For this review, take the finished solid that the model builds, in its own axes (mm). A direction names the side the tool comes from. Round coordinates to 2 decimals unless told otherwise and drop trailing zeros. Order: outer loops, then holes, each group sorted by start corner. A loop starts at its lowest first (then second) coordinate and runs counter-clockwise, first axis right, second up. Notation, with made-up numbers: (73.5, -4.75) -> (86.5, -4.75) arc R31 cw to (86.5, 25.25) -> close; hole circle Ø3 at (-23.75, 2.5). An arc over 180 degrees is marked (long way). Answer in a Markdown table with one row per item.
```python
from build123d import *

# Parameters (mm, degrees)
CROQUIS1_W               = 16.7
CROQUIS1_H               = 20.1
SALIENTE_EXTRUIR1_DEPTH  = 3.2
CROQUIS2_W               = 20
CROQUIS2_H               = 3.2
SALIENTE_EXTRUIR2_DEPTH  = 16.7
SALIENTE_EXTRUIR3_DEPTH  = 2.2
SALIENTE_EXTRUIR4_DEPTH  = 2.2
CROQUIS5_W               = 6.7
CROQUIS5_H               = 2.4
CORTAR_EXTRUIR1_DEPTH    = 3.2
CROQUIS6_W               = 6.7
CROQUIS6_H               = 2.3
CORTAR_EXTRUIR2_DEPTH    = 3.2
CROQUIS7_W               = 4.1
CROQUIS7_H               = 1.18
SALIENTE_EXTRUIR9_DEPTH  = 1.45
SALIENTE_EXTRUIR10_DEPTH = 4.1
CROQUIS10_W              = 4.098890586
CROQUIS10_H              = 1.18
SALIENTE_EXTRUIR13_DEPTH = 1.45
SALIENTE_EXTRUIR14_DEPTH = 4.1
SALIENTE_EXTRUIR16_DEPTH = 4.1


with BuildPart() as part:
    # Croquis1 → Saliente-Extruir1 (new body)
    with BuildSketch(Plane.XY):
        Rectangle(CROQUIS1_W, CROQUIS1_H)
    extrude(amount=SALIENTE_EXTRUIR1_DEPTH)

    # Croquis2 → Saliente-Extruir2 (add)
    with BuildSketch(Plane.ZY.offset(8.35)):
        with Locations((10, 8.45)):
            Rectangle(CROQUIS2_W, CROQUIS2_H)
    extrude(amount=-SALIENTE_EXTRUIR2_DEPTH)

    # Croquis3 → Saliente-Extruir3 (add)
    with BuildSketch(Plane.ZY.offset(8.35)):
        Polygon((20, 6.85), (3.2, -10.05), (3.2, 6.85), align=None)
    extrude(amount=-SALIENTE_EXTRUIR3_DEPTH)

    # Croquis4 → Saliente-Extruir4 (add)
    with BuildSketch(Plane(origin=(8.35, 0, 0), x_dir=(0, 0, -1), z_dir=(1, 0, 0))):
        Polygon((-20, 6.85), (-3.2, -10.05), (-3.2, 6.85), align=None)
    extrude(amount=-SALIENTE_EXTRUIR4_DEPTH)

    # Croquis5 → Cortar-Extruir1 (cut)
    with BuildSketch(Plane(origin=(0, 0, 0), x_dir=(-1, 0, 0), z_dir=(0, 0, -1))):
        with BuildLine():
            ThreePointArc((-3.35, 1.5), (0, 4.85), (3.35, 1.5))
            Line((3.35, 1.5), (-3.35, 1.5))
        make_face()
        with Locations((0, 0.3)):
            Rectangle(CROQUIS5_W, CROQUIS5_H)
        with BuildLine():
            Line((3.35, -0.9), (-3.35, -0.9))
            ThreePointArc((-3.35, -0.9), (0, -4.25), (3.35, -0.9))
        make_face()
    extrude(amount=-CORTAR_EXTRUIR1_DEPTH, mode=Mode.SUBTRACT)

    # Croquis6 → Cortar-Extruir2 (cut)
    with BuildSketch(Plane(origin=(0, 10.05, 0), x_dir=(1, 0, 0), z_dir=(0, 1, 0))):
        with BuildLine():
            ThreePointArc((-3.35, -9.15), (0, -5.8), (3.35, -9.15))
            Line((3.35, -9.15), (-3.35, -9.15))
        make_face()
        with Locations((0, -10.3)):
            Rectangle(CROQUIS6_W, CROQUIS6_H)
        with BuildLine():
            Line((3.35, -11.45), (-3.35, -11.45))
            ThreePointArc((-3.35, -11.45), (0, -14.8), (3.35, -11.45))
        make_face()
    extrude(amount=-CORTAR_EXTRUIR2_DEPTH, mode=Mode.SUBTRACT)

    # Croquis7 → Saliente-Extruir9 (add)
    with BuildSketch(Plane(origin=(0, 0, 0), x_dir=(-1, 0, 0), z_dir=(0, 0, -1))):
        with Locations((0, 7.46)):
            Rectangle(CROQUIS7_W, CROQUIS7_H)
        with Locations((0, -7.34)):
            Rectangle(CROQUIS7_W, CROQUIS7_H)
    extrude(amount=SALIENTE_EXTRUIR9_DEPTH)

    # Croquis9 → Saliente-Extruir10 (add)
    with BuildSketch(Plane.ZY.offset(2.05)):
        Polygon((-1.45, 6.87), (0, 5.75), (0, 6.87), align=None)
        Polygon((-1.45, -7.93), (0, -9.05), (0, -7.93), align=None)
    extrude(amount=-SALIENTE_EXTRUIR10_DEPTH)

    # Croquis10 → Saliente-Extruir13 (add)
    with BuildSketch(Plane(origin=(0, 10.05, 0), x_dir=(1, 0, 0), z_dir=(0, 1, 0))):
        with Locations((-0.000554707, -2.59)):
            Rectangle(CROQUIS10_W, CROQUIS10_H)
        with Locations((-0.000554707, -17.29)):
            Rectangle(CROQUIS10_W, CROQUIS10_H)
    extrude(amount=SALIENTE_EXTRUIR13_DEPTH)

    # Croquis12 → Saliente-Extruir14 (add)
    with BuildSketch(Plane(origin=(2.048890586, 0, 0), x_dir=(0, 0, -1), z_dir=(1, 0, 0))):
        Polygon((-17.88, 11.5), (-19, 10.05), (-17.88, 10.05), align=None)
        Polygon((-3.18, 11.5), (-4.3, 10.05), (-3.18, 10.05), align=None)
    extrude(amount=-SALIENTE_EXTRUIR14_DEPTH)

    # Croquis13 → Saliente-Extruir16 (add)
    with BuildSketch(Plane.ZY.offset(2.05)):
        Polygon((2, 11.5), (2, 10.05), (4.3, 10.05), (3.18, 11.5), align=None)
        Polygon((16.7, 11.5), (16.7, 10.05), (19, 10.05), (17.88, 11.5), align=None)
    extrude(amount=-SALIENTE_EXTRUIR16_DEPTH)


solid = part.part
```
Q1. Take a section at C-C, the plane z = 0.5. Write out the cut boundary in (x, y).
Answer key:
| item | result |
|---|---|
| outline | (-8.35, -10.05) -> (8.35, -10.05) -> (8.35, 10.05) -> (-8.35, 10.05) -> close; hole (-3.35, -0.9) arc R3.35 ccw to (3.35, -0.9) -> (3.35, 1.5) arc R3.35 ccw to (-3.35, 1.5) -> close |
Q2. The part is to be moulded in two halves that separate along X. For faces 4 (the face through (-7.3, -1.5, 11.7)), 5 (the face through (-2.051, 10.5, 18.2)), 6 (the face through (0, 6.85, 15)), 7 (the face through (3.35, 0, 2)), say which applies: +X half, -X half, draft (parallel to the pull), parting line (faces both ways), or undercut.
Answer key:
| item | result |
|---|---|
| face 4 | draft |
| face 5 | -X half |
| face 6 | undercut |
| face 7 | undercut |
Q3. Take a section at B-B, the plane y = 9.5. Write out the cut boundary in (x, z).
Answer key:
| item | result |
|---|---|
| outline | (-8.35, 0) -> (8.35, 0) -> (8.35, 20) -> (-8.35, 20) -> close; hole (-3.35, 9.15) arc R3.35 ccw to (3.35, 9.15) -> (3.35, 11.45) arc R3.35 ccw to (-3.35, 11.45) -> close |
Q4. Tool access review of faces 1 (the face through (2.05, 11, 3)), 2 (the face through (-2.05, 11, 17)), 3 (the face through (0, 11, 16.7)): name each direction out of +Z, -Z, +X, -X, +Y, -Y from which nothing blocks a thin tool from reaching the whole face with its end or side.
Answer key:
| item | result |
|---|---|
| face 1 | +Z, -Z, +X, +Y |
| face 2 | +Z, -Z, -X, +Y |
| face 3 | +X, -X, +Y |
Q5. Take a section at A-A, the plane x = 0. Give the number of separate pieces and of enclosed holes in the cut face, then the cut area to 3 significant figures.
Answer key:
| item | result |
|---|---|
| separate pieces | 3 |
| enclosed holes | 0 |
| area | 70.3 mm^2 |
Q6. To check wall thickness, follow probe 1 along X at (y, z) = (0, 6); probe 2 along Z at (x, y) = (2, -5.5); probe 3 along X at (y, z) = (7, 6.25). State the ranges of each line that lie inside material, in increasing order.
Answer key:
| item | result |
|---|---|
| probe 1 | x = -8.35 to -6.15, 6.15 to 8.35 |
| probe 2 | z = 0 to 3.2 |
| probe 3 | x = -8.35 to -1.68, 1.68 to 8.35 |
Q7. Clearance check with flat-ended pins moving along their axes: pin 1 Ø1.5 at (x, z) = (-4, 3.5) entering from -Y; pin 2 Ø6 at (x, y) = (-2.5, 0) entering from +Z; pin 3 Ø6 at (x, z) = (-1.5, 7.5) entering from -Y; pin 4 Ø1.3 at (y, z) = (11, 3) entering from -X. State where each tip first meets the part, or that it passes through.
Answer key:
| item | result |
|---|---|
| pin 1 | stops at y = -10.05 |
| pin 2 | stops at z = 3.2 |
| pin 3 | stops at y = 6.85 |
| pin 4 | stops at x = -2.05 |
Q8. Take a section at D-D, the plane y = -3.75. Write out the cut boundary in (x, z), then the cut area to 3 significant figures.
Answer key:
| item | result |
|---|---|
| outline | (-8.35, 0) -> (-1.76, 0) -> (-1.76, 3.2) -> (-6.15, 3.2) -> (-6.15, 9.46) -> (-8.35, 9.46) -> close; (1.76, 0) -> (8.35, 0) -> (8.35, 9.46) -> (6.15, 9.46) -> (6.15, 3.2) -> (1.76, 3.2) -> close |
| area | 69.7 mm^2 |
